The model under review builds one solid part; all positions refer to its coordinate system, in mm. A direction names the side the tool comes from. Round coordinates to 2 decimals unless told otherwise and drop trailing zeros. Loops run counter-clockwise (first coordinate to the right, second up) from the corner with the lowest first, then second, coordinate; pieces in that order, holes last. Notation, with made-up numbers: M 25,76.5 L 46,76.5 A21 ccw 46,91.5 Z; hole C 37.25,5 d11. An arc over 180 degrees is marked long. Return JSON: item names as keys, results as strings. Group by question number.
Q1. Draft analysis for pull direction X (two halves, no side actions). For faces 4 (the face through (-6.662, -21.328, 7.395)), 5 (the face through (22.85, -6.4, 7.4)), 6 (the face through (0, 0, 15)), state which applies: pulls with the +X half, pulls with the -X half, needs draft (parallel to the pull), parting line crosses it, or undercut.
Q2. Consider section C-C (z = 3). State the section outline as (x, y) points.
Q3. To check wall thickness, follow line 1 along Y through (x, z) = (21.5, 13); line 2 along X through (y, z) = (4, 5.25); line 3 along X through (y, z) = (21, 5.25). State the ranges of each line that lie inside material, in increasing order.
Q4. Consider section A-A (z = 7.5). State the section outline as (x, y) points.
Q5. Clearance check with flat-ended pins moving along their axes: pin 1 Ø2 at (x, z) = (5, 7.5) entering from -Y; pin 2 Ø6 at (y, z) = (-16.5, 10.5) entering from +X; pin 3 Ø2 at (y, z) = (-25, 6) entering from +X; pin 4 Ø12 at (x, y) = (8, 4) entering from -Z. State where each tip first meets the part, or that it passes through.
Q6. Consider section D-D (y = -8). State the section outline as (x, z) points, and give its area (3 significant figures).
Q7. Consider section B-B (x = 0). State the section outline as (y, z) points.
Q8. For faces 1 (the face through (-7.5, -24, 7)), 2 (the face through (2, 12, 5)), 3 (the face through (-19.722, 21.507, 7.395)), list the 3-axis set-ups (+Z, -Z, +X, -X, +Y, -Y) from which the entire face can be reached by the end or side of a thin tool; tool diameter is ignored.
from build123d import *

# Parameters (mm, degrees)
SZKIC1_R                    = 2.25
DODANIE_WYCI_GNI_CIE1_DEPTH = 15
SZKIC2_R                    = 16
SZKIC2_R_2                  = 12
WYTNIJ_WYCI_GNI_CIE1_DEPTH  = 10


with BuildPart() as part:
    # Szkic1 → Dodanie-wyciągnięcie1 (new body)
    with BuildSketch(Plane.XY):
        with BuildLine():
            Line((-7.5, -25.4), (-27.5000055, -25.4))
            Line((-27.5000055, -25.4), (-27.5000055, 0))
            ThreePointArc((-27.5000055, 0), (-26.360400157, 7.560626052), (-23.04284729, 14.449429258))
            ThreePointArc((-23.04284729, 14.449429258), (-22.876506159, 15.134411684), (-23.203344978, 15.75894886))
            Line((-23.203344978, 15.75894886), (-25.196922194, 17.537575813))
            ThreePointArc((-25.196922194, 17.537575813), (-25.467611983, 22.191093586), (-20.814747272, 22.472785982))
            Line((-20.814747272, 22.472785982), (-18.598905377, 20.514600122))
            ThreePointArc((-18.598905377, 20.514600122), (-17.974550182, 20.264645495), (-17.333078903, 20.466663618))
            ThreePointArc((-17.333078903, 20.466663618), (9.576401492, 22.98111988), (23.8, 0))
            ThreePointArc((23.8, 0), (22.82107067, -6.492449946), (19.979075206, -12.411340949))
            ThreePointArc((19.979075206, -12.411340949), (19.813964518, -13.098271951), (20.143734708, -13.723081814))
            Line((20.143734708, -13.723081814), (22.185252728, -15.527214018))
            ThreePointArc((22.185252728, -15.527214018), (22.472785982, -20.185252728), (17.814747272, -20.472785982))
            Line((17.814747272, -20.472785982), (15.376980036, -18.318480053))
            ThreePointArc((15.376980036, -18.318480053), (14.777726241, -18.069792078), (14.151976117, -18.241220202))
            ThreePointArc((14.151976117, -18.241220202), (4.948796089, -21.832347138), (-4.899043329, -21.048271831))
            ThreePointArc((-4.899043329, -21.048271831), (-6.68281162, -21.343100938), (-7.5, -22.955849111))
            Line((-7.5, -22.955849111), (-7.5, -25.4))
        make_face()
        with Locations((-23, 20)):
            Circle(SZKIC1_R, mode=Mode.SUBTRACT)
        with Locations((20, -18)):
            Circle(SZKIC1_R, mode=Mode.SUBTRACT)
    extrude(amount=DODANIE_WYCI_GNI_CIE1_DEPTH)

    # Szkic2 → Wytnij-wyciągnięcie1 (cut)
    with BuildSketch(Plane.XY.offset(15)):
        Circle(SZKIC2_R)
        Circle(SZKIC2_R_2, mode=Mode.SUBTRACT)
    extrude(amount=-WYTNIJ_WYCI_GNI_CIE1_DEPTH, mode=Mode.SUBTRACT)


solid = part.part
Values:
{
 "1": {"face 4": "undercut", "face 5": "pulls with the +X half", "face 6": "needs draft"},
 "2": {"outline": "M -27.5,-25.4 L -7.5,-25.4 L -7.5,-22.96 A2 cw -4.9,-21.05 A22.07 ccw 14.15,-18.24 A1 cw 15.38,-18.32 L 17.81,-20.47 A3.3 ccw 22.19,-15.53 L 20.14,-13.72 A1 cw 19.98,-12.41 A22.12 ccw 23.8,0 A25.65 ccw -17.33,20.47 A1 cw -18.6,20.51 L -20.81,22.47 A3.3 ccw -25.2,17.54 L -23.2,15.76 A1 cw -23.04,14.45 A25.65 ccw -27.5,0 Z; hole C -23,20 d4.5; hole C 20,-18 d4.5"},
 "3": {"line 1": "y = -20.94 to -19.68, -16.32 to -14.92, -9.81 to 10.63", "line 2": "x = -27.19 to -15.49, -11.31 to 11.31, 15.49 to 23.49", "line 3": "x = -26.14 to -25.02, -20.98 to -19.15, -16.6 to 12.9"},
 "4": {"outline": "M -27.5,-25.4 L -7.5,-25.4 L -7.5,-22.96 A2 cw -4.9,-21.05 A22.07 ccw 14.15,-18.24 A1 cw 15.38,-18.32 L 17.81,-20.47 A3.3 ccw 22.19,-15.53 L 20.14,-13.72 A1 cw 19.98,-12.41 A22.12 ccw 23.8,0 A25.65 ccw -17.33,20.47 A1 cw -18.6,20.51 L -20.81,22.47 A3.3 ccw -25.2,17.54 L -23.2,15.76 A1 cw -23.04,14.45 A25.65 ccw -27.5,0 Z; C 0,0 d24; hole C -23,20 d4.5; hole C 0,0 d32; hole C 20,-18 d4.5"},
 "5": {"pin 1": "stops at y = -21.95", "pin 2": "stops at x = 23.3", "pin 3": "stops at x = -7.5", "pin 4": "stops at z = 0"},
 "6": {"outline": "M -27.5,0 L 22.3,0 L 22.3,15 L 13.86,15 L 13.86,5 L 8.94,5 L 8.94,15 L -8.94,15 L -8.94,5 L -13.86,5 L -13.86,15 L -27.5,15 Z", "area": "649 mm2"},
 "7": {"outline": "M -22,0 L 25.6,0 L 25.6,15 L 16,15 L 16,5 L 12,5 L 12,15 L -12,15 L -12,5 L -16,5 L -16,15 L -22,15 Z"},
 "8": {"face 1": "+Z, -Z, +X, -Y", "face 2": "+Z", "face 3": "+Z, -Z, +Y"}
}
